The figure shows three views and two pictorial views of one solid part (mm, origin at its lowest corner). Answer the questions. Give positions to 0.01 mm unless a question says otherwise; leave off trailing zeros. Order: outer loops, then holes, each group sorted by start corner. A loop starts at its lowest first (then second) coordinate and runs counter-clockwise, first axis right, second up. Notation, with made-up numbers: (89, 22.25) - (104, 22.25) arc R18 cw to (104, 46.25) - close; hole circle Ø5 at (-2, 6). An arc over 180 degrees is marked (long way). Use a Markdown table: item, result. Add a question column.
1. A flat-ended cylindrical pin translates along its axis: P1, Ø3, axis at x = 66.24, z = 85.64, coming from the -Y side. Find the tip coordinate at first contact, or state that the pin passes through.
2. A cutting plane is placed at B-B on y = 0.75. Determine the outline of the cut face in (x, z), and give its area (3 significant figures).
3. A cutting plane is placed at A-A on x = 80. Determine the outline of the cut face in (y, z).
4. Consider L1, parallel to Z at x = 99, y = 2.4; L2, parallel to X at y = 0.9, z = 77.5. Determine where each line is inside the solid, lowest interval first.
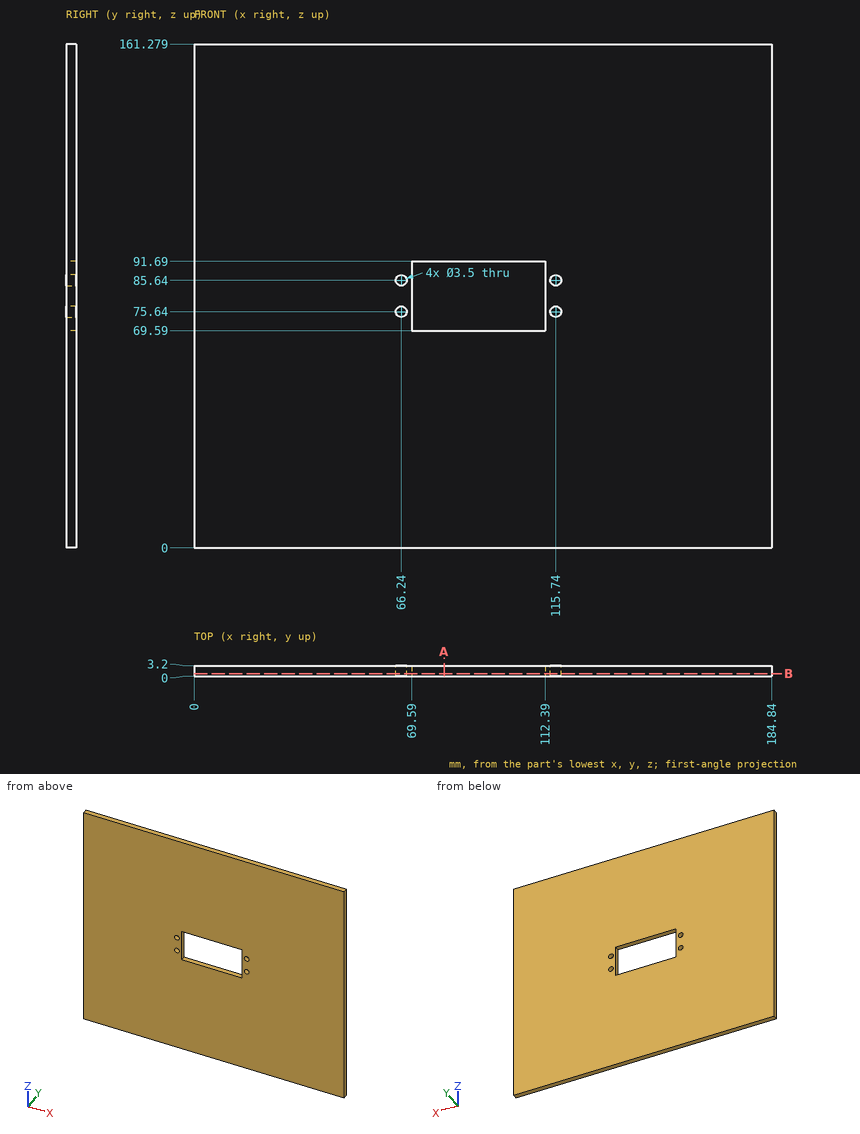
Output values:
| question | item | result |
|---|---|---|
| 1 | P1 | through |
| 2 | outline | (0, 0) - (184.84, 0) - (184.84, 161.28) - (0, 161.28) - close; hole circle Ø3.5 at (66.24, 75.64); hole circle Ø3.5 at (66.24, 85.64); hole (69.59, 69.59) - (112.39, 69.59) - (112.39, 91.69) - (69.59, 91.69) - close; hole circle Ø3.5 at (115.74, 75.64); hole circle Ø3.5 at (115.74, 85.64) |
| 2 | area | 28,800 mm² |
| 3 | outline | (0, 0) - (3.2, 0) - (3.2, 69.59) - (0, 69.59) - close; (0, 91.69) - (3.2, 91.69) - (3.2, 161.28) - (0, 161.28) - close |
| 4 | L1 | 0 to 69.59, 91.69 to 161.28 |
| 4 | L2 | 0 to 69.59, 112.39 to 184.84 |
